Check sheet for the modelled part. Datum: model origin and axes. Units: mm. Face numbers are marked on the shaded views. A direction names the side the tool comes from. Give positions to 0.01 mm unless a question says otherwise; leave off trailing zeros. Write each loop counter-clockwise with the first axis right and the second up, starting at its lowest first coordinate (ties: lowest second). Pieces come first, ordered by that corner, then holes. Notation, with made-up numbers: (-19, 30) -> (18, 30) arc R15 cw to (18, 38) -> close; hole circle Ø4 at (89, 64.5). An arc over 180 degrees is marked (long way). Return JSON: item names as keys, results as strings.
from build123d import *

# Parameters (mm, degrees)
SKETCH1_W           = 42.3
SKETCH1_H           = 42.3
BOSS_EXTRUDE1_DEPTH = 34
FILLET1_SIZE        = 7
SKETCH1_3_R         = 1.5
CUT_EXTRUDE1_DEPTH  = 4
SKETCH3_R           = 11
SKETCH3_R_2         = 2.5
BOSS_EXTRUDE2_DEPTH = 2
SKETCH3_2_R         = 2.5
BOSS_EXTRUDE3_DEPTH = 24
CHAMFER1_SIZE       = 0.2


with BuildPart() as part:
    # Sketch1 → Boss-Extrude1 (new body)
    with BuildSketch(Plane(origin=(0, 0, 0), x_dir=(1, 0, 0), z_dir=(0, 1, 0))):
        Rectangle(SKETCH1_W, SKETCH1_H)
    extrude(amount=-BOSS_EXTRUDE1_DEPTH)

    # Fillet1
    # a fillet whose section is not a circle: 7 mm, written as the material it takes off along each edge
    with BuildSketch(Plane(origin=(21.15, 17.5, 21.15), x_dir=(-1, 0, 0), z_dir=(0, -1, 0)), Plane(origin=(21.15, 17.5, -21.15), x_dir=(0, 0, 1), z_dir=(0, -1, 0)), Plane(origin=(-21.15, 17.5, -21.15), x_dir=(1, 0, 0), z_dir=(0, -1, 0))) as fillet1_piece_1:
        with BuildLine():
            Bezier((FILLET1_SIZE, 0), (0, 0), (0, FILLET1_SIZE), weights=[1, 0.333333333, 1])
            Line((0, FILLET1_SIZE), (0, 0))
            Line((0, 0), (FILLET1_SIZE, 0))
        make_face()
    extrude(amount=69, mode=Mode.SUBTRACT)
    with BuildSketch(Plane(origin=(-21.15, 17.5, 21.15), x_dir=(1, 0, 0), z_dir=(0, -1, 0))) as fillet1_piece_2:
        with BuildLine():
            Bezier((FILLET1_SIZE, 0), (0, 0), (0, -FILLET1_SIZE), weights=[1, 0.333333333, 1])
            Line((0, -FILLET1_SIZE), (0, 0))
            Line((0, 0), (FILLET1_SIZE, 0))
        make_face()
    extrude(amount=69, mode=Mode.SUBTRACT)

    # Sketch1<3> → Cut-Extrude1 (cut)
    with BuildSketch(Plane(origin=(0, 0, 0), x_dir=(1, 0, 0), z_dir=(0, 1, 0))):
        with Locations(Location((-15.55, -15.55, 0), (0, 0, 270))):
            Circle(SKETCH1_3_R)
        with Locations(Location((-15.55, 15.55, 0), (0, 0, 270))):
            Circle(SKETCH1_3_R)
        with Locations(Location((15.55, 15.55, 0), (0, 0, 270))):
            Circle(SKETCH1_3_R)
        with Locations(Location((15.55, -15.55, 0), (0, 0, 270))):
            Circle(SKETCH1_3_R)
    extrude(amount=-CUT_EXTRUDE1_DEPTH, mode=Mode.SUBTRACT)

    # Sketch3 → Boss-Extrude2 (add)
    with BuildSketch(Plane(origin=(0, 0, 0), x_dir=(1, 0, 0), z_dir=(0, 1, 0))):
        with Locations(Location((0, 0, 0), (0, 0, 270))):
            Circle(SKETCH3_R)
        with Locations(Location((0, 0, 0), (0, 0, 270))):
            Circle(SKETCH3_R_2, mode=Mode.SUBTRACT)
    extrude(amount=BOSS_EXTRUDE2_DEPTH)

    # Sketch3<2> → Boss-Extrude3 (add)
    with BuildSketch(Plane(origin=(0, 0, 0), x_dir=(1, 0, 0), z_dir=(0, 1, 0))):
        with Locations(Location((0, 0, 0), (0, 0, 270))):
            Circle(SKETCH3_2_R)
    extrude(amount=BOSS_EXTRUDE3_DEPTH)

    # Chamfer1
    chamfer1_edges = [part.edges().sort_by_distance(p)[0] for p in [
        (0, 24, -2.5),
    ]]
    chamfer(chamfer1_edges, length=CHAMFER1_SIZE)


solid = part.part
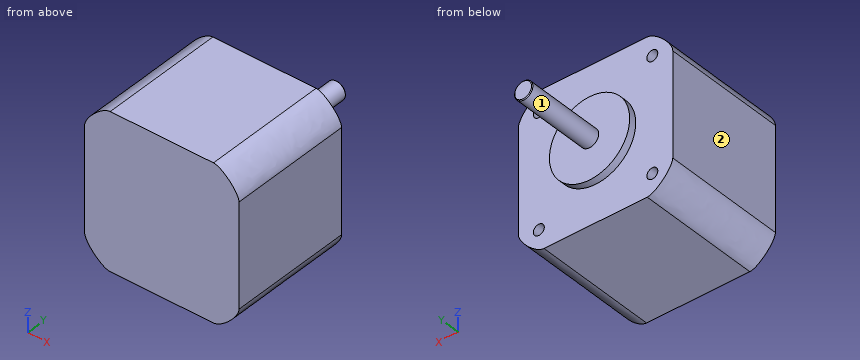
(1) Depth check by flat-ended pin: pin 1 Ø3.5 at (x, z) = (16, 16) entering from +Y; pin 2 Ø1.5 at (x, z) = (-16, 16) entering from +Y. Enter the tip coordinate at first touch or a pass-through.
Reply:
{"pin 1": "y = 0", "pin 2": "y = -4"}
(2) Cross-section at B-B on x = 0. Enter the section's corners in (y, z), then the cut area to 3 significant figures.
Reply:
{"outline": "(-34, -21.15) -> (0, -21.15) -> (0, -11) -> (2, -11) -> (2, -2.5) -> (23.8, -2.5) -> (24, -2.3) -> (24, 2.3) -> (23.8, 2.5) -> (2, 2.5) -> (2, 11) -> (0, 11) -> (0, 21.15) -> (-34, 21.15) -> close", "area": "1,590 mm^2"}
(3) Cross-section at C-C on y = 7. Enter the section's corners in (x, z), then the cut area to 3 significant figures.
Reply:
{"outline": "circle Ø5 at (0, 0)", "area": "19.6 mm^2"}
(4) Thickness scan on L1, parallel to X at y = -2.9, z = 15.55; L2, parallel to Y at x = -17, z = 3; L3, parallel to Y at x = 15.5, z = 16. Record the ranges inside material, lowest first.
Reply:
{"L1": "-20.75 to -17.05, -14.05 to 14.05, 17.05 to 20.75", "L2": "-34 to 0", "L3": "-34 to -4"}
(5) Cross-section at A-A on z = 0. Enter the section's corners in (x, y).
Reply:
{"outline": "(-21.15, -34) -> (21.15, -34) -> (21.15, 0) -> (11, 0) -> (11, 2) -> (2.5, 2) -> (2.5, 23.8) -> (2.3, 24) -> (-2.3, 24) -> (-2.5, 23.8) -> (-2.5, 2) -> (-11, 2) -> (-11, 0) -> (-21.15, 0) -> close"}
(6) Set-up check for the marked faces 1 and 2: record each of +Z, -Z, +X, -X, +Y, -Y from which the full face is reachable in a straight line by a thin tool's end or side.
Reply:
{"face 1": "+Y", "face 2": "+Z, -Z, -X, +Y, -Y"}
(7) Cross-section at D-D on z = -6. Enter the section's corners in (x, y), then the cut area to 3 significant figures.
Reply:
{"outline": "(-21.15, -34) -> (21.15, -34) -> (21.15, 0) -> (9.22, 0) -> (9.22, 2) -> (-9.22, 2) -> (-9.22, 0) -> (-21.15, 0) -> close", "area": "1,480 mm^2"}
